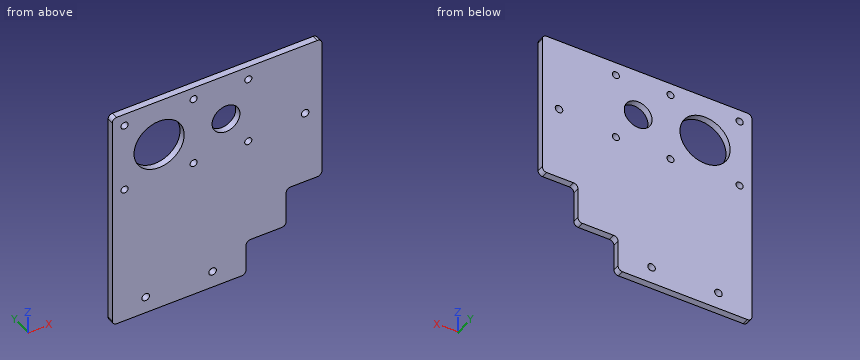
Autodesk Inventor part; units mm, degrees
ref_plane "YZ Plane" through (0, 0, 0) normal (1, 0, 0) x (0, 1, 0)
ref_plane "XZ Plane" through (0, 0, 0) normal (0, 1, 0) x (-1, 0, 0)
ref_plane "XY Plane" through (0, 0, 0) normal (0, 0, 1) x (1, 0, 0)
sketch "Sketch1" plane through (0, 0, 0) normal (0, 1, 0) x (-1, 0, 0)
  line L0 (0, 34) -> (0, 100)
  line L1 (0, 100) -> (94, 100)
  line L2 (94, 100) -> (94, 0)
  line L3 (94, 0) -> (34, 0)
  circle A0 centre (57.5, 94.5) radius 1.6
  circle A1 centre (88.5, 94.5) radius 1.6
  circle A2 centre (88.5, 63.5) radius 1.6
  circle A3 centre (57.5, 63.5) radius 1.6
  circle A4 centre (73, 79) radius 11.25
  circle A5 centre (43, 79) radius 6.25
  line L4 (34, 16) -> (16, 16)
  line L5 (16, 16) -> (16, 34)
  line L6 (34, 0) -> (34, 16)
  line L7 (16, 34) -> (0, 34)
  circle A6 centre (33, 64) radius 1.6
  circle A7 centre (33, 94) radius 1.6
  point P0 (0, 0)
  dimension "d3" = 100
  dimension "d4" = 60
  dimension "d5" = 31
  dimension "d6" = 31
  dimension "d7" = 15.5
  dimension "d8" = 15.5
  dimension "d9" = 22.5
  dimension "d10" = 21
  dimension "d11" = 12.5
  dimension "d12" = 21
  dimension "d13" = 3.2
  dimension "d14" = 30
  dimension "d15" = 16
  dimension "d16" = 34
  dimension "d17" = 34
  dimension "d18" = 15
  dimension "d19" = 15
  dimension "d20" = 10
extrude "Extrusion1" add sketch "Sketch1" along normal blind 3
fillet "Fillet1" radius 2 8 edges at (-16, 1.5, 34) (-34, 1.5, 16) (-16, 1.5, 16) (0, 1.5, 34) (-34, 1.5, 0) (0, 1.5, 100) (-94, 1.5, 100) (-94, 1.5, 0)
sketch "Sketch2" plane through (0, 0, 0) normal (0, -1, 0) x (1, 0, 0)
  arc A0 (-94, 2) -> (-92, 0) centre (-92, 2) ccw
  line L0 (-36, 0) -> (-92, 0)
  arc A1 (-36, 0) -> (-34, 2) centre (-36, 2) ccw
  line L1 (-34, 14) -> (-34, 2)
  arc A2 (-32, 16) -> (-34, 14) centre (-32, 14) ccw
  line L2 (-18, 16) -> (-32, 16)
  arc A3 (-18, 16) -> (-16, 18) centre (-18, 18) ccw
  line L3 (-16, 32) -> (-16, 18)
  arc A4 (-14, 34) -> (-16, 32) centre (-14, 32) ccw
  line L4 (-2, 34) -> (-14, 34)
  arc A5 (-2, 34) -> (0, 36) centre (-2, 36) ccw
  line L5 (0, 98) -> (0, 36)
  arc A6 (0, 98) -> (-2, 100) centre (-2, 98) ccw
  line L6 (-92, 100) -> (-2, 100)
  arc A7 (-92, 100) -> (-94, 98) centre (-92, 98) ccw
  line L7 (-94, 2) -> (-94, 98)
  circle A8 centre (-33, 94) radius 1.6
  circle A9 centre (-33, 64) radius 1.6
  circle A10 centre (-43, 79) radius 6.25
  circle A11 centre (-73, 79) radius 11.25
  circle A12 centre (-57.5, 63.5) radius 1.6
  circle A13 centre (-88.5, 63.5) radius 1.6
  circle A14 centre (-88.5, 94.5) radius 1.6
  circle A15 centre (-57.5, 94.5) radius 1.6
  point P0 (0, 0)
  point P1 (-7.5, 67)
  point P2 (-49, 7.5)
  point P3 (-79, 7.5)
  point P4 (0, 67)
  dimension "d22" = 7.5
  dimension "d23" = 7.5
  dimension "d24" = 15
  dimension "d25" = 15
hole "Hole1" at (-7.5, 0, 67) at (-49, 0, 7.5) at (-79, 0, 7.5) direction (0, 1, 0) diameter 3.4 end through all
equation "\"d6\" = d5"
equation "\"d7\" = 0.5 * d6"
equation "\"d8\" = 0.5 * d5"
equation "\"d19\" = d18"
properties part number "Z Axis Motor Mount" material "Aluminum 6061"
Input: part model. Units: mm. Frame: model coordinates. Give positions to 0.01 mm unless a question says otherwise; leave off trailing zeros. Order: outer loops, then holes, each group sorted by start corner. A loop starts at its lowest first (then second) coordinate and runs counter-clockwise, first axis right, second up.
Q1. Contact query for a flat-ended pin moving along its axis: pin 1 Ø0.9 at (x, y) = (-25, 2) entering from -Z. Output: stop coordinate, or through.
Checked values:
pin 1: stops at z = 16
Q2. Section A-A on x = -7.5. Output: boundary loops of the cut face in (y, z).
Checked values:
outline: (0, 34) - (3, 34) - (3, 65.3) - (0, 65.3) - close; (0, 68.7) - (3, 68.7) - (3, 100) - (0, 100) - close
Q3. Section D-D on x = -43. Output: boundary loops of the cut face in (y, z), and give its area (4 significant figures).
Checked values:
outline: (0, 0) - (3, 0) - (3, 72.75) - (0, 72.75) - close; (0, 85.25) - (3, 85.25) - (3, 100) - (0, 100) - close
area: 262.5 mm2
Q4. Section C-C on x = -88.5. Output: boundary loops of the cut face in (y, z).
Checked values:
outline: (0, 0) - (3, 0) - (3, 61.9) - (0, 61.9) - close; (0, 65.1) - (3, 65.1) - (3, 92.9) - (0, 92.9) - close; (0, 96.1) - (3, 96.1) - (3, 100) - (0, 100) - close
Q5. Section B-B on z = 7.5. Output: boundary loops of the cut face in (x, y).
Checked values:
outline: (-94, 0) - (-80.7, 0) - (-80.7, 3) - (-94, 3) - close; (-77.3, 0) - (-50.7, 0) - (-50.7, 3) - (-77.3, 3) - close; (-47.3, 0) - (-34, 0) - (-34, 3) - (-47.3, 3) - close
Q6. Ray query, probe 1 along Z at (x, y) = (-43.5, 1.55); probe 2 along Z at (x, y) = (-57.5, 0.4); probe 3 along X at (y, z) = (1.7, 7.5). Return the intervals inside material, ascending.
Checked values:
probe 1: z = 0 to 72.77, 85.23 to 100
probe 2: z = 0 to 61.9, 65.1 to 92.9, 96.1 to 100
probe 3: x = -94 to -80.7, -77.3 to -50.7, -47.3 to -34
